```python
from build123d import *

# Parameters (mm, degrees)
F0_W     = 38.1
F0_H     = 5.08
F1_DEPTH = 7.62
F3_T     = -1.27


# Not quite as in the source:
# - a feature of the source that left no trace in its solid (it failed there, or was rolled back) is left out


with BuildPart() as f1:
    # F0 (on Front) → F1 (new body)
    with BuildSketch(Plane.XZ):
        with Locations((-46.2881572708, 42.3315375688)):
            Rectangle(F0_W, F0_H)
    extrude(amount=F1_DEPTH)

    # F3
    f3_openings = [f1.faces().sort_by_distance(p)[0] for p in [
        (-46.288157, -7.62, 42.331538),
    ]]
    offset(amount=F3_T, openings=f3_openings)


solid = f1.part
```
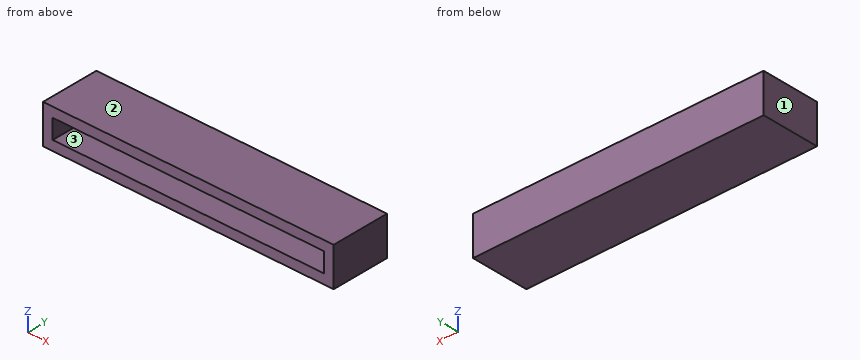
Build history of the part. All positions in model axes, mm. Face numbers are marked on the shaded views. Give positions to 0.01 mm unless a question says otherwise; leave off trailing zeros. Loops run counter-clockwise (first coordinate to the right, second up) from the corner with the lowest first, then second, coordinate; pieces in that order, holes last.
1) Band-saw the part on B-B on x = -47. List the corners of the cut face in (y, z).
Values follow:
outline: (-7.62, 39.79) - (0, 39.79) - (0, 44.87) - (-7.62, 44.87) - (-7.62, 43.6) - (-1.27, 43.6) - (-1.27, 41.06) - (-7.62, 41.06) - close
2) Band-saw the part on A-A on y = -6. List the corners of the cut face in (x, z).
Values follow:
outline: (-65.34, 39.79) - (-27.24, 39.79) - (-27.24, 44.87) - (-65.34, 44.87) - close; hole (-64.07, 41.06) - (-28.51, 41.06) - (-28.51, 43.6) - (-64.07, 43.6) - close
3) Band-saw the part on C-C on z = 42.35. List the corners of the cut face in (x, y).
Values follow:
outline: (-65.34, -7.62) - (-64.07, -7.62) - (-64.07, -1.27) - (-28.51, -1.27) - (-28.51, -7.62) - (-27.24, -7.62) - (-27.24, 0) - (-65.34, 0) - close
4) Probe line 1 along Z through (x, y) = (-47, -7); line 2 along X through (y, z) = (-5.75, 42.4); line 3 along Y through (x, z) = (-58, 41.85). List the from-to ranges inside material, lowest first.
Values follow:
line 1: z = 39.79 to 41.06, 43.6 to 44.87
line 2: x = -65.34 to -64.07, -28.51 to -27.24
line 3: y = -1.27 to 0
5) Two-plate mould, pull along Z, no slides. Class the marked faces 1, 2 and 3: released by +Z, released by -Z, zero draft, split by the parting line, or undercut.
Values follow:
face 1: zero draft
face 2: released by +Z
face 3: undercut
